Check sheet for the modelled part. Datum: model origin and axes. Units: mm. Face numbers are marked on the shaded views. A direction names the side the tool comes from. Coordinates: 2 decimals unless noted, no trailing zeros. Loops run counter-clockwise (first coordinate to the right, second up) from the corner with the lowest first, then second, coordinate; pieces in that order, holes last. Notation, with made-up numbers: M -31.75,-35.5 L -21.75,-35.5 A15 cw -21.75,-18.5 Z; hole C 9.5,70 d4. An arc over 180 degrees is marked long. Return JSON: item names as keys, results as strings.
Autodesk Inventor part; units mm, degrees
ref_plane "Work Plane1" through (0, 0, 150) normal (0, 0, 1) x (1, 0, 0)
ref_plane "Work Plane2" through (-18.5938, -147.8125, 150) normal (1, 0, 0) x (0, 0, -1)
ref_plane "YZ Plane" through (0, 0, 0) normal (1, 0, 0) x (0, 1, 0)
sketch "Sketch1" plane through (0, 0, 0) normal (0, 0, 1) x (1, 0, 0)
  line L0 (-368.5938, -273.4375) -> (-368.5938, 352.1875)
  line L1 (-368.5938, 352.1875) -> (331.4062, 352.1875)
  line L2 (331.4062, 352.1875) -> (331.4062, -247.8125)
  line L3 (331.4062, -247.8125) -> (-368.5938, -247.8125)
  line L4 (-368.5938, -247.8125) -> (-368.5938, -273.4375)
  point P0 (0, 0)
  dimension "d0" = 700
  dimension "d1" = 600
extrude "Extrusion1" add sketch "Sketch1" along normal blind 150
ref_plane "Work Plane1" through (0, 0, 150) normal (0, 0, 1) x (1, 0, 0)
sketch "Sketch2" plane through (0, 0, 150) normal (0, 0, 1) x (1, 0, 0)
  line L0 (-268.5938, -147.8125) -> (-268.5938, 252.1875)
  line L1 (-268.5938, 252.1875) -> (231.4062, 252.1875)
  line L2 (231.4062, 252.1875) -> (231.4063, -147.8125)
  line L3 (231.4063, -147.8125) -> (-268.5938, -147.8125)
  line L4 (331.4062, 352.1875) -> (-368.5938, 352.1875)
  line L5 (331.4062, -247.8125) -> (331.4062, 352.1875)
  point P0 (0, 0)
  dimension "d5" = 500
  dimension "d6" = 400
  dimension "d7" = 100
  dimension "d8" = 100
extrude "Extrusion2" add sketch "Sketch2" along normal blind 100
sketch "Sketch3" plane through (231.4062, -147.8125, 150) normal (1, 0, 0) x (0, 0, -1)
  line L0 (-100, 0) -> (-100, 400)
  line L1 (-100, 0) -> (-250, 0)
  line L2 (-350, 100) -> (-350, 300)
  line L3 (-250, 400) -> (-100, 400)
  line L4 (0, 400) -> (-100, 400)
  line L5 (-250, 400) -> (-350, 300)
  line L6 (-250, 0) -> (-350, 100)
  point P0 (150, 147.8125)
  point P1 (-350, 0)
  point P2 (-350, 400)
  dimension "d11" = 250
  dimension "d12" = 400
  dimension "d13" = 100
  dimension "d14" = 45
  dimension "d15" = 100
  dimension "d16" = 45
extrude "Extrusion3" add sketch "Sketch3" against normal blind 150
ref_plane "Work Plane2" through (-18.5938, -147.8125, 150) normal (1, 0, 0) x (0, 0, -1)
mirror "Mirror1" about plane through (-18.5938, -147.8125, 150) normal (1, 0, 0) of "Extrusion3"
equation "\"d16\" = d14"
properties part number "BT020_Doppelführung"
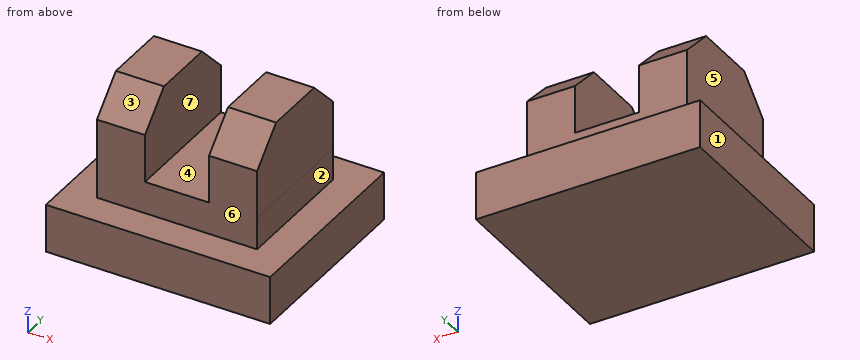
1) Section check B-B on x = 100.5. Record the cut outline in (y, z).
Answers:
{"outline": "M -247.81,0 L 352.19,0 L 352.19,150 L 252.19,150 L 252.19,400 L 152.19,500 L -47.81,500 L -147.81,400 L -147.81,150 L -247.81,150 Z"}
2) Go/stop test with flat-tipped pins: pin 1 Ø10 at (x, z) = (231, 283) entering from +Y; pin 2 Ø12 at (y, z) = (212, 195) entering from +X; pin 3 Ø6 at (x, z) = (153, 179.5) entering from -Y. Record where each tip stops, or that it passes through.
Answers:
{"pin 1": "y = 252.19", "pin 2": "x = 231.41", "pin 3": "y = -147.81"}
3) Section check D-D on z = 190.5. Record the cut outline in (x, y), then the cut area to 3 significant figures.
Answers:
{"outline": "M -268.59,-147.81 L 231.41,-147.81 L 231.41,252.19 L -268.59,252.19 Z", "area": "200,000 mm²"}
4) Draft check along X on the marked faces 1, 2, 3 and 4. Enter one of: +X half, -X half, draft (parallel to the pull), parting line (faces both ways), or undercut.
Answers:
{"face 1": "-X half", "face 2": "+X half", "face 3": "draft", "face 4": "undercut"}
5) Section check A-A on z = 268.5. Record the cut outline in (x, y).
Answers:
{"outline": "M -268.59,-147.81 L -118.59,-147.81 L -118.59,252.19 L -268.59,252.19 Z; M 81.41,-147.81 L 231.41,-147.81 L 231.41,252.19 L 81.41,252.19 Z"}
6) Set-up check for the marked faces 5, 6 and 7: record each of +Z, -Z, +X, -X, +Y, -Y from which the full face is reachable in a straight line by a thin tool's end or side.
Answers:
{"face 5": "+Z, -X, +Y, -Y", "face 6": "+Z, +X, -X, -Y", "face 7": "+Z, +Y, -Y"}
7) Scan lines: line 1 along X through (y, z) = (-51, 396); line 2 along Y through (x, z) = (-6, 233.5); line 3 along Z through (x, y) = (-73.5, 8). Record each from-to range of solid material in increasing order. Write a range as [from, to].
Answers:
{"line 1": "[-268.59, -118.59], [81.41, 231.41]", "line 2": "[-147.81, 252.19]", "line 3": "[0, 250]"}
